Here's how the part is built. I have some questions about the finished solid (model axes, mm). A direction names the side the tool comes from. Round coordinates to 2 decimals unless told otherwise and drop trailing zeros. Write each loop counter-clockwise with the first axis right and the second up, starting at its lowest first coordinate (ties: lowest second). Pieces come first, ordered by that corner, then holes. Notation, with made-up numbers: (-8, -28) -> (30, -28) arc R28 cw to (30, -6) -> close; hole circle Ø4 at (-9.75, -11.75). An arc over 180 degrees is marked (long way). Put each result on its own line as item: value. Start each with the question number.
1) I want a section at A-A, the plane z = -13. Give the number of separate pieces and of enclosed holes in the cut face, then the cut area to 3 significant figures.
2) I want a section at C-C, the plane y = 0. List the corners of the cut face in (x, z) for me, then the cut area to 3 significant figures.
3) Which directions (+Z, -Z, +X, -X, +Y, -Y) give clear straight access to the entire face, cutting with the end or side of a thin tool? Please do faces 1 (the cylindrical face through (-15.729, -26.984, -12.867)), 2 (the flat face through (14.75, -17, -15)).
4) If I drill on line 1 along X through (y, z) = (-21.5, -13.5); line 2 along Z through (x, y) = (8.25, -36.1) (3 decimals); line 3 along Y through (x, z) = (16.2, -25) (3 decimals), over which ranges is the centre line in solid material (lowest first)? Write a range as [from, to].
5) Will these pins go through, and if not, where does the flat tip stop? P1, Ø8, axis at x = -3.5, z = -24.5, coming from the +Y side; P2, Ø14.5, axis at x = 5.5, y = -23, coming from the -Z side.
6) I want a section at B-B, the plane x = -7.75. List the corners of the cut face in (y, z) for me (3 decimals), then the cut area to 3 significant figures.
7) We'd pull the mould along Z, two halves only. Please class faces 3 (the cylindrical face through (8.117, -36.771, -23.984)), 4 (the cylindrical face through (0.47, -37.68, 2.4)), 5 (the cylindrical face through (-16.68, -37.65, -14.28)): released by +Z, released by -Z, zero draft, split by the parting line, or undercut.
from build123d import *

# Parameters (mm, degrees)
EXTRUDE_1_DEPTH     = 3
EXTRUDE_2_DEPTH     = 30
SKETCH_3_R          = 1.025
CUT_EXTRUDE_1_DEPTH = 43
SKETCH_4_R          = 1.025
CUT_EXTRUDE_2_DEPTH = 3
FILLET_1_R          = 2


with BuildPart() as part:
    # Sketch 2 → Extrude 1 (new body)
    with BuildSketch(Plane.XY):
        with BuildLine():
            ThreePointArc((-9.721835338, 0.75), (0.25, -10), (10.221835338, 0.75))
            Line((10.221835338, 0.75), (14.75, 0.75))
            Line((14.75, 0.75), (14.75, -35.25))
            Line((14.75, -35.25), (-14.25, -35.25))
            Line((-14.25, -35.25), (-14.25, 0.75))
            Line((-14.25, 0.75), (-9.721835338, 0.75))
        make_face()
        Polygon((-14.25, -35.25), (-14.25, 0.75), (-17.25, 0.75), (-17.25, -38.25), (17.75, -38.25), (17.75, 0.75), (14.75, 0.75), (14.75, -35.25), align=None)
    extrude(amount=EXTRUDE_1_DEPTH)

    # Sketch 2_6 → Extrude 2 (add)
    with BuildSketch(Plane.XY):
        Polygon((-14.25, -35.25), (-14.25, 0.75), (-17.25, 0.75), (-17.25, -38.25), (17.75, -38.25), (17.75, 0.75), (14.75, 0.75), (14.75, -35.25), align=None)
    extrude(amount=-EXTRUDE_2_DEPTH)

    # Sketch 3 → Cut-Extrude 1 (cut)
    with BuildSketch(Plane(origin=(17.75, 0, 0), x_dir=(0, 0, -1), z_dir=(1, 0, 0))):
        with Locations((25, -4)):
            Circle(SKETCH_3_R)
        with Locations((13, -4)):
            Circle(SKETCH_3_R)
        with Locations((25, -28)):
            Circle(SKETCH_3_R)
        with Locations((13, -28)):
            Circle(SKETCH_3_R)
    extrude(amount=-CUT_EXTRUDE_1_DEPTH, mode=Mode.SUBTRACT)

    # Sketch 4 → Cut-Extrude 2 (cut)
    with BuildSketch(Plane.XZ.offset(38.25)):
        with Locations((8.25, -25)):
            Circle(SKETCH_4_R)
        with Locations((-7.75, -25)):
            Circle(SKETCH_4_R)
        with Locations((-7.75, -13)):
            Circle(SKETCH_4_R)
        with Locations((8.25, -13)):
            Circle(SKETCH_4_R)
    extrude(amount=-CUT_EXTRUDE_2_DEPTH, mode=Mode.SUBTRACT)

    # Fillet 1
    fillet_1_edges = [part.edges().sort_by_distance(p)[0] for p in [
        (-17.25, -18.75, 3),
        (17.75, -38.25, -13.5),
        (-17.25, -38.25, -13.5),
        (0.25, -38.25, 3),
        (17.75, -18.75, 3),
    ]]
    fillet(fillet_1_edges, radius=FILLET_1_R)


solid = part.part
Findings:
1. separate pieces: 7
1. enclosed holes: 0
1. area: 282 mm2
2. outline: (-17.25, -30) -> (-14.25, -30) -> (-14.25, 0) -> (-9.75, 0) -> (-9.75, 3) -> (-15.25, 3) arc R2 ccw to (-17.25, 1) -> close; (10.25, 0) -> (14.75, 0) -> (14.75, -30) -> (17.75, -30) -> (17.75, 1) arc R2 ccw to (15.75, 3) -> (10.25, 3) -> close
2. area: 223 mm2
3. face 1: +X, -X
3. face 2: -Z, +Y
4. line 1: x = [-17.25, -14.25], [14.75, 17.75]
4. line 2: z = [-30, -26.025], [-23.975, -14.025], [-11.975, 3]
4. line 3: y = [-38.199, -29.025], [-26.975, -5.025], [-2.975, 0.75]
5. P1: stops at y = -35.25
5. P2: stops at z = 0
6. outline: (-38.25, -30) -> (-35.25, -30) -> (-35.25, -26.025) -> (-38.25, -26.025) -> close; (-38.25, -23.975) -> (-35.25, -23.975) -> (-35.25, -14.025) -> (-38.25, -14.025) -> close; (-38.25, -11.975) -> (-35.25, -11.975) -> (-35.25, 0) -> (-6, 0) -> (-6, 3) -> (-36.25, 3) arc R2 ccw to (-38.25, 1) -> close
6. area: 174 mm2
7. face 3: undercut
7. face 4: released by +Z
7. face 5: zero draft
